Build history of the part. All positions in model axes, mm. A direction names the side the tool comes from. Round coordinates to 2 decimals unless told otherwise and drop trailing zeros. Write each loop counter-clockwise with the first axis right and the second up, starting at its lowest first coordinate (ties: lowest second). Pieces come first, ordered by that corner, then holes. Notation, with made-up numbers: M 15.5,-33.5 L 30.5,-33.5 A12 cw 30.5,-19.5 Z; hole C 67,55.5 d1. An arc over 180 degrees is marked long. Use a Markdown table: item, result.
from build123d import *

# Parameters (mm, degrees)
F3_R     = 1.5
F4_DEPTH = 14.001


with BuildPart() as f1:
    # F0 (on Front) → F1 (revolve)
    with BuildSketch(Plane.XZ):
        Polygon((-7, 6.5), (-7, -7.5), (-6.2, -7.5), (-4.75, -3.516158), (-4.75, 2.5), (0, 6.5), (0, 7.5), (-6.25, 7.5), (-6.25, 6.5), align=None)
    revolve(axis=Axis((0, 0, 0.727193), (0, 0, -1)))

    # F3 (on offset) → F4 (cut, through all)
    with BuildSketch(Plane.XZ.offset(7)):
        Circle(F3_R)
    extrude(amount=-F4_DEPTH, mode=Mode.SUBTRACT)


solid = f1.part
Q1. Two-plate mould, pull along Z, no slides. Class faces 4 (the cylindrical face through (-1.5, -5.77, 0.07)), 5 (the cylindrical face through (-5.96, 1.88, 6.99)), 6 (the conical face through (0.16, -0.74, 5.86)): +Z half, -Z half, draft (parallel to the pull), parting line (faces both ways), or undercut.
Response values:
| item | result |
|---|---|
| face 4 | undercut |
| face 5 | draft |
| face 6 | -Z half |
Q2. Cut at D-D on z = -5.75. Give the cut face in (x, y), and give its area (3 significant figures).
Response values:
| item | result |
|---|---|
| outline | C 0,0 d14; hole C 0,0 d11.13 |
| area | 56.7 mm2 |
Q3. Cut at B-B on z = -4. Give the cut face in (x, y), and give its area (3 significant figures).
Response values:
| item | result |
|---|---|
| outline | C 0,0 d14; hole C 0,0 d9.85 |
| area | 77.7 mm2 |
Q4. Cut at C-C on x = 1. Count the separate pieces of the cut face and the enclosed holes in it, and give its area (3 significant figures).
Response values:
| item | result |
|---|---|
| separate pieces | 3 |
| enclosed holes | 0 |
| area | 80.7 mm2 |
Q5. Drop flat-ended pins along their axis: P1, Ø2, axis at x = 4.5, z = 1.5, coming from the +Y side; P2, Ø1, axis at y = -4, z = 6, coming from the +X side; P3, Ø2, axis at x = 2.5, z = -5, coming from the +Y side. Give the stop position or say it passes through.
Response values:
| item | result |
|---|---|
| P1 | stops at y = 6.06 |
| P2 | stops at x = 6.06 |
| P3 | stops at y = 6.84 |
Q6. Cut at A-A on z = 0. Give the cut face in (x, y), and give its area (3 significant figures).
Response values:
| item | result |
|---|---|
| outline | M -1.5,-6.84 L -1.5,-4.51 A4.75 cw -1.5,4.51 L -1.5,6.84 A7 ccw Z; M 1.5,-6.84 A7 ccw 1.5,6.84 L 1.5,4.51 A4.75 cw 1.5,-4.51 Z |
| area | 69.4 mm2 |
Q7. Drill centre lines: L1, parallel to X at y = -5.25, z = 0; L2, parallel to Z at x = 0, y = -6.4; L3, parallel to Y at x = -1.75, z = -4.5. Where is each one in solid material? Low to high.
Response values:
| item | result |
|---|---|
| L1 | x = -4.63 to -1.5, 1.5 to 4.63 |
| L2 | z = -7.5 to -1.5, 1.5 to 6.5 |
| L3 | y = -6.78 to -4.8, 4.8 to 6.78 |
Q8. Which spindle directions (+Z, -Z, +X, -X, +Y, -Y) get a long thin tool onto all of the face, cutting with end or side? Do faces 1 (the flat face through (4, -5, -7.5)), 2 (the cylindrical face through (-4.388, -1.819, -0.466)), 3 (the flat face through (-3, 6, 6.5)). Say none if no direction does.
Response values:
| item | result |
|---|---|
| face 1 | -Z, +X, -X, +Y, -Y |
| face 2 | -Z |
| face 3 | +Z |
